Part model, mm, in its own coordinate system. A direction names the side the tool comes from. Give positions to 0.01 mm unless a question says otherwise; leave off trailing zeros. Order: outer loops, then holes, each group sorted by start corner. A loop starts at its lowest first (then second) coordinate and runs counter-clockwise, first axis right, second up. Notation, with made-up numbers: M 11.5,-34.5 L 51.5,-34.5 A23 ccw 51.5,-4.5 Z; hole C 36,-6 d5. An arc over 180 degrees is marked long. Return JSON: item names as keys, results as strings.
from build123d import *

# Parameters (mm, degrees)
SKETCH1_W               = 104
SKETCH1_H               = 153
BOSS_EXTRUDE1_DEPTH     = 10
CUT_EXTRUDE1_DEPTH      = 156.226704492
CUT_EXTRUDE1_DEPTH_BACK = 156.226704492
SKETCH2_W               = 84
SKETCH2_H               = 133
CUT_EXTRUDE3_DEPTH      = 156.226704492
CUT_EXTRUDE3_DEPTH_BACK = 156.226704492
SKETCH3_W               = 10
SKETCH3_H               = 97
FILLET9_R               = 5
FILLET10_R              = 5
FILLET11_R              = 5
FILLET12_R              = 5


with BuildPart() as part:
    # Sketch1 → Boss-Extrude1 (new body)
    with BuildSketch(Plane.XY):
        with Locations((25.638107417, -57.543478261)):
            Rectangle(SKETCH1_W, SKETCH1_H)
    extrude(amount=BOSS_EXTRUDE1_DEPTH)

    # Sketch2 → Cut-Extrude1 (cut, two sides: drawn at the far end of the back side and taken through both)
    with BuildSketch(Plane.XY.offset(10).offset(-CUT_EXTRUDE1_DEPTH_BACK)):
        with Locations((25.638107417, -57.543478261)):
            Rectangle(SKETCH2_W, SKETCH2_H)
    extrude(amount=CUT_EXTRUDE1_DEPTH + CUT_EXTRUDE1_DEPTH_BACK, mode=Mode.SUBTRACT)

    # Sketch3 → Cut-Extrude3 (cut, two sides: drawn at the far end of the back side and taken through both)
    with BuildSketch(Plane.XY.offset(10).offset(-CUT_EXTRUDE3_DEPTH_BACK)):
        with Locations((72.638107417, -57.543478261)):
            Rectangle(SKETCH3_W, SKETCH3_H)
    extrude(amount=CUT_EXTRUDE3_DEPTH + CUT_EXTRUDE3_DEPTH_BACK, mode=Mode.SUBTRACT)

    # Fillet9
    fillet9_edges = [part.edges().sort_by_distance(p)[0] for p in [
        (-16.361892583, 8.956521739, 5),
    ]]
    fillet(fillet9_edges, radius=FILLET9_R)

    # Fillet10
    fillet10_edges = [part.edges().sort_by_distance(p)[0] for p in [
        (67.638107417, 8.956521739, 5),
        (-26.361892583, 18.956521739, 5),
    ]]
    fillet(fillet10_edges, radius=FILLET10_R)

    # Fillet11
    fillet11_edges = [part.edges().sort_by_distance(p)[0] for p in [
        (67.638107417, -124.043478261, 5),
        (77.638107417, 18.956521739, 5),
        (-26.361892583, -134.043478261, 5),
    ]]
    fillet(fillet11_edges, radius=FILLET11_R)

    # Fillet12
    fillet12_edges = [part.edges().sort_by_distance(p)[0] for p in [
        (-16.361892583, -124.043478261, 5),
        (77.638107417, -134.043478261, 5),
    ]]
    fillet(fillet12_edges, radius=FILLET12_R)


solid = part.part
Q1. Probe line 1 along Y through (x, z) = (25, 5); line 2 along X through (y, z) = (-111, 3); line 3 along X through (y, z) = (-27.5, 5.75). List the from-to ranges inside material, lowest first.
Established:
{"line 1": "y = -134.04 to -124.04, 8.96 to 18.96", "line 2": "x = -26.36 to -16.36, 67.64 to 77.64", "line 3": "x = -26.36 to -16.36"}
Q2. 3-axis set-ups, long thin cutter, end or side, ignore diameter. For faces 1 (the flat face through (25, -124.043, 5)), 2 (the flat face through (-17, -57, 10)), 3 (the flat face through (73, -106.043, 5)): which of +Z, -Z, +X, -X, +Y, -Y reach the whole face in a straight line?
Established:
{"face 1": "+Z, -Z", "face 2": "+Z, +X, -X, +Y, -Y", "face 3": "+Z, -Z, +X"}
Q3. Band-saw the part on A-A (y = -112). Give the cut face in (x, z), then the cut area to 3 significant figures.
Established:
{"outline": "M -26.36,0 L -16.36,0 L -16.36,10 L -26.36,10 Z; M 67.64,0 L 77.64,0 L 77.64,10 L 67.64,10 Z", "area": "200 mm²"}
Q4. Band-saw the part on C-C (z = 5.75). Give the cut face in (x, y).
Established:
{"outline": "M -26.36,-129.04 A5 ccw -21.36,-134.04 L 72.64,-134.04 A5 ccw 77.64,-129.04 L 77.64,-106.04 L 67.64,-106.04 L 67.64,-119.04 A5 cw 62.64,-124.04 L -11.36,-124.04 A5 cw -16.36,-119.04 L -16.36,3.96 A5 cw -11.36,8.96 L 62.64,8.96 A5 cw 67.64,3.96 L 67.64,-9.04 L 77.64,-9.04 L 77.64,13.96 A5 ccw 72.64,18.96 L -21.36,18.96 A5 ccw -26.36,13.96 Z"}
Q5. Band-saw the part on D-D (y = -65.5). Give the cut face in (x, z), then the cut area to 3 significant figures.
Established:
{"outline": "M -26.36,0 L -16.36,0 L -16.36,10 L -26.36,10 Z", "area": "100 mm²"}
Q6. Pin check, flat tip, straight feed: pin 1 (3 mm diameter, centred on x = 74, z = 5, fed in from +Y). Stop position of the tip, or through.
Established:
{"pin 1": "stops at y = 18.96"}
Q7. Band-saw the part on B-B (x = 42.5). Give the cut face in (y, z).
Established:
{"outline": "M -134.04,0 L -124.04,0 L -124.04,10 L -134.04,10 Z; M 8.96,0 L 18.96,0 L 18.96,10 L 8.96,10 Z"}
Q8. Two-plate mould, pull along Y, no slides. Class faces 4 (the flat face through (-16.362, -58, 5)), 5 (the cylindrical face through (-24.936, -132.54, 5.07)), 6 (the flat face through (77.638, -118, 5)): +Y half, -Y half, draft (parallel to the pull), parting line (faces both ways), or undercut.
Established:
{"face 4": "undercut", "face 5": "-Y half", "face 6": "draft"}
